Job drawing, mm, ordinate dimensions from the low corner. One solid piece. A direction names the side the tool comes from. Give positions to 0.01 mm unless a question says otherwise; leave off trailing zeros. Order: outer loops, then holes, each group sorted by start corner. A loop starts at its lowest first (then second) coordinate and runs counter-clockwise, first axis right, second up.
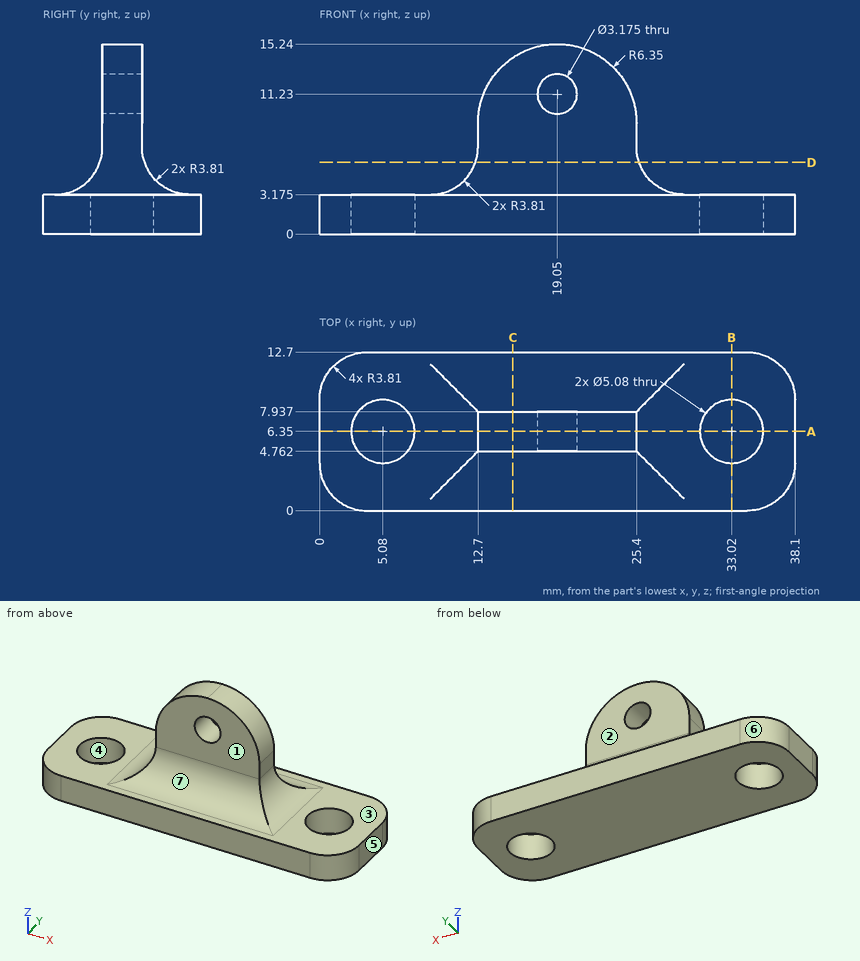
Item 1: Band-saw the part on D-D on z = 5.75. List the corners of the cut face in (x, y) (1 decimal).
Item 2: Pull direction Y, two halves, no side cores. Call the marked faces 4, 5, 6 and 7: released by +Y, released by -Y, zero draft, split by the parting line, or undercut.
Item 3: Band-saw the part on B-B on x = 33.02. List the corners of the cut face in (y, z) (1 decimal).
Item 4: Which spindle directions (+Z, -Z, +X, -X, +Y, -Y) get a long thin tool onto all of the face, cutting with end or side? Do the marked faces 1, 2 and 3. Say none if no direction does.
Item 5: Band-saw the part on A-A on y = 6.35. Give the number of separate pieces and of enclosed holes in the cut face, plus the area to 3 significant figures.
Item 6: Drop flat-ended pins along their axis: P1, Ø5, axis at x = 27.5, y = 9, coming from the -Z side; P2, Ø4, axis at x = 19.05, z = 11.23, coming from the +Y side; P3, Ø3, axis at y = 5, z = 7, coming from the +X side; P4, Ø3, axis at x = 8.5, y = 10, coming from the +Z side. Give the stop position or say it passes through.
Item 7: Band-saw the part on C-C on x = 15.5. List the corners of the cut face in (y, z) (1 decimal).
Item 8: Drill centre lines: probe 1 along Z at (x, y) = (19.05, 7.1); probe 2 along Y at (x, z) = (33.02, 0.7); probe 3 along Z at (x, y) = (25, 0.5) (1 decimal). Where is each one in solid material? Low to high.
Working result:
1. outline: (12.5, 4.6) - (25.6, 4.6) - (25.6, 8.1) - (12.5, 8.1) - close
2. face 4: undercut
2. face 5: zero draft
2. face 6: released by +Y
2. face 7: released by -Y
3. outline: (0, 0) - (3.8, 0) - (3.8, 3.2) - (0, 3.2) - close; (8.9, 0) - (12.7, 0) - (12.7, 3.2) - (8.9, 3.2) - close
4. face 1: +Z, +X, -X, -Y
4. face 2: +Z, +X, -X, +Y
4. face 3: +Z
5. separate pieces: 3
5. enclosed holes: 1
5. area: 223 mm2
6. P1: stops at z = 0
6. P2: stops at y = 7.94
6. P3: stops at x = 25.7
6. P4: stops at z = 3.34
7. outline: (0, 0) - (12.7, 0) - (12.7, 3.2) - (11.7, 3.2) arc R3.8 cw to (7.9, 7) - (7.9, 14.2) - (4.8, 14.2) - (4.8, 7) arc R3.8 cw to (1, 3.2) - (0, 3.2) - close
8. probe 1: z = 0 to 9.64, 12.82 to 15.24
8. probe 2: y = 0 to 3.81, 8.89 to 12.7
8. probe 3: z = 0 to 3.2
